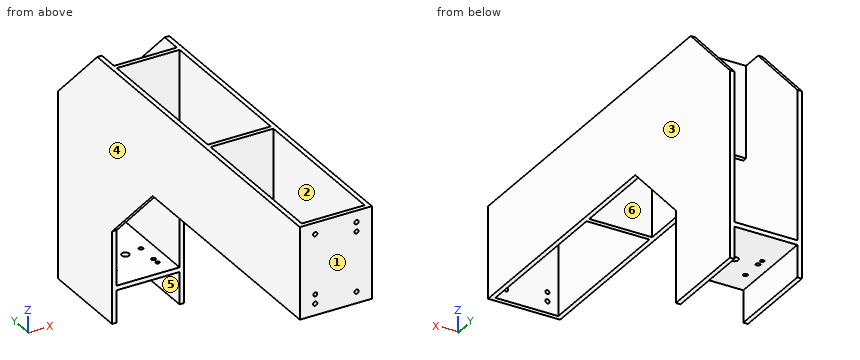
```python
from build123d import *

# Parameters (mm, degrees)
BOSS_EXTRUDE1_DEPTH      = 10
BOSS_EXTRUDE1_DEPTH_BACK = 147
SKETCH3_W                = 137
SKETCH3_H                = 550
CUT_EXTRUDE1_DEPTH       = 885
SKETCH4_W                = 137
SKETCH4_H                = 200
BOSS_EXTRUDE2_DEPTH      = 10
CUT_EXTRUDE3_REACH       = 82
SKETCH6_R                = 4.5
SKETCH6_R_2              = 8
SKETCH6_R_3              = 4.25
SKETCH8_W                = 157
SKETCH8_H                = 200
BOSS_EXTRUDE3_DEPTH      = 10
LPATTERN1_COUNT          = 3
LPATTERN1_PITCH          = 347.5
CUT_EXTRUDE4_REACH       = 12
SKETCH7_R                = 4.5
SKETCH7_R_2              = 4.25


with BuildPart() as part:
    # Sketch1 → Boss-Extrude1 (new body, two sides)
    with BuildSketch(Plane(origin=(0, 0, 0), x_dir=(0, 0, -1), z_dir=(1, 0, 0))) as boss_extrude1_sk:
        Polygon((200, 695), (200, 545), (350, 695), align=None)
        Polygon((200, 0), (200, 695), (550, 695), (550, 895), (145, 895), (0, 750), (0, 0), align=None)
    extrude(amount=BOSS_EXTRUDE1_DEPTH)
    extrude(boss_extrude1_sk.sketch, amount=-BOSS_EXTRUDE1_DEPTH_BACK)

    # Sketch3 → Cut-Extrude1 (cut)
    with BuildSketch(Plane(origin=(0, 895, 0), x_dir=(1, 0, 0), z_dir=(0, 1, 0))):
        with Locations((-68.5, 275)):
            Rectangle(SKETCH3_W, SKETCH3_H)
    extrude(amount=-CUT_EXTRUDE1_DEPTH, mode=Mode.SUBTRACT)

    # Sketch4 → Boss-Extrude2 (add)
    with BuildSketch(Plane(origin=(0, 0, -480), x_dir=(-1, 0, 0), z_dir=(0, 0, -1))):
        with Locations((68.5, 795)):
            Rectangle(SKETCH4_W, SKETCH4_H)
    extrude(amount=-BOSS_EXTRUDE2_DEPTH)

    # Sketch6 → Cut-Extrude3 (cut, up to next)
    with BuildSketch(Plane.XY.offset(-470), mode=Mode.PRIVATE) as cut_extrude3_sk1:
        with Locations((-111, 747.2)):
            Circle(SKETCH6_R)
    cut_extrude3_tool1 = extrude(cut_extrude3_sk1.sketch, amount=-CUT_EXTRUDE3_REACH, mode=Mode.PRIVATE) & part.part
    add(cut_extrude3_tool1.solids().sort_by_distance((-111, 747.2, -470))[0], mode=Mode.SUBTRACT)
    # Sketch6 → Cut-Extrude3 (cut, up to next)
    with BuildSketch(Plane.XY.offset(-470), mode=Mode.PRIVATE) as cut_extrude3_sk2:
        with Locations((-26, 747.2)):
            Circle(SKETCH6_R)
    cut_extrude3_tool2 = extrude(cut_extrude3_sk2.sketch, amount=-CUT_EXTRUDE3_REACH, mode=Mode.PRIVATE) & part.part
    add(cut_extrude3_tool2.solids().sort_by_distance((-26, 747.2, -470))[0], mode=Mode.SUBTRACT)
    # Sketch6 → Cut-Extrude3 (cut, up to next)
    with BuildSketch(Plane.XY.offset(-470), mode=Mode.PRIVATE) as cut_extrude3_sk3:
        with Locations((-111, 793.7)):
            Circle(SKETCH6_R)
    cut_extrude3_tool3 = extrude(cut_extrude3_sk3.sketch, amount=-CUT_EXTRUDE3_REACH, mode=Mode.PRIVATE) & part.part
    add(cut_extrude3_tool3.solids().sort_by_distance((-111, 793.7, -470))[0], mode=Mode.SUBTRACT)
    # Sketch6 → Cut-Extrude3 (cut, up to next)
    with BuildSketch(Plane.XY.offset(-470), mode=Mode.PRIVATE) as cut_extrude3_sk4:
        with Locations((-26, 793.7)):
            Circle(SKETCH6_R)
    cut_extrude3_tool4 = extrude(cut_extrude3_sk4.sketch, amount=-CUT_EXTRUDE3_REACH, mode=Mode.PRIVATE) & part.part
    add(cut_extrude3_tool4.solids().sort_by_distance((-26, 793.7, -470))[0], mode=Mode.SUBTRACT)
    # Sketch6 → Cut-Extrude3 (cut, up to next)
    with BuildSketch(Plane.XY.offset(-470), mode=Mode.PRIVATE) as cut_extrude3_sk5:
        with Locations((-63, 788.5)):
            Circle(SKETCH6_R_2)
    cut_extrude3_tool5 = extrude(cut_extrude3_sk5.sketch, amount=-CUT_EXTRUDE3_REACH, mode=Mode.PRIVATE) & part.part
    add(cut_extrude3_tool5.solids().sort_by_distance((-63, 788.5, -470))[0], mode=Mode.SUBTRACT)
    # Sketch6 → Cut-Extrude3 (cut, up to next)
    with BuildSketch(Plane.XY.offset(-470), mode=Mode.PRIVATE) as cut_extrude3_sk6:
        with Locations((-111, 808.7)):
            Circle(SKETCH6_R_3)
    cut_extrude3_tool6 = extrude(cut_extrude3_sk6.sketch, amount=-CUT_EXTRUDE3_REACH, mode=Mode.PRIVATE) & part.part
    add(cut_extrude3_tool6.solids().sort_by_distance((-111, 808.7, -470))[0], mode=Mode.SUBTRACT)
    # Sketch6 → Cut-Extrude3 (cut, up to next)
    with BuildSketch(Plane.XY.offset(-470), mode=Mode.PRIVATE) as cut_extrude3_sk7:
        with Locations((-26, 732.2)):
            Circle(SKETCH6_R_3)
    cut_extrude3_tool7 = extrude(cut_extrude3_sk7.sketch, amount=-CUT_EXTRUDE3_REACH, mode=Mode.PRIVATE) & part.part
    add(cut_extrude3_tool7.solids().sort_by_distance((-26, 732.2, -470))[0], mode=Mode.SUBTRACT)

    # Sketch8 → Boss-Extrude3 (add)
    with BuildSketch(Plane(origin=(0, 705, 0), x_dir=(-1, 0, 0), z_dir=(0, -1, 0))):
        with Locations((68.5, 100)):
            Rectangle(SKETCH8_W, SKETCH8_H)
    boss_extrude3 = extrude(amount=BOSS_EXTRUDE3_DEPTH)

    # LPattern1: Boss-Extrude3 ×3
    with Locations(*[(0, -i * LPATTERN1_PITCH, 0) for i in range(1, LPATTERN1_COUNT)]):
        add(boss_extrude3)

    # Sketch7 → Cut-Extrude4 (cut, up to next)
    with BuildSketch(Plane(origin=(0, 10, 0), x_dir=(1, 0, 0), z_dir=(0, 1, 0)), mode=Mode.PRIVATE) as cut_extrude4_sk1:
        with Locations((-113.5, 175)):
            Circle(SKETCH7_R)
    cut_extrude4_tool1 = extrude(cut_extrude4_sk1.sketch, amount=-CUT_EXTRUDE4_REACH, mode=Mode.PRIVATE) & part.part
    add(cut_extrude4_tool1.solids().sort_by_distance((-113.5, 10, -175))[0], mode=Mode.SUBTRACT)
    # Sketch7 → Cut-Extrude4 (cut, up to next)
    with BuildSketch(Plane(origin=(0, 10, 0), x_dir=(1, 0, 0), z_dir=(0, 1, 0)), mode=Mode.PRIVATE) as cut_extrude4_sk2:
        with Locations((-23.5, 175)):
            Circle(SKETCH7_R)
    cut_extrude4_tool2 = extrude(cut_extrude4_sk2.sketch, amount=-CUT_EXTRUDE4_REACH, mode=Mode.PRIVATE) & part.part
    add(cut_extrude4_tool2.solids().sort_by_distance((-23.5, 10, -175))[0], mode=Mode.SUBTRACT)
    # Sketch7 → Cut-Extrude4 (cut, up to next)
    with BuildSketch(Plane(origin=(0, 10, 0), x_dir=(1, 0, 0), z_dir=(0, 1, 0)), mode=Mode.PRIVATE) as cut_extrude4_sk3:
        with Locations((-23.5, 25)):
            Circle(SKETCH7_R)
    cut_extrude4_tool3 = extrude(cut_extrude4_sk3.sketch, amount=-CUT_EXTRUDE4_REACH, mode=Mode.PRIVATE) & part.part
    add(cut_extrude4_tool3.solids().sort_by_distance((-23.5, 10, -25))[0], mode=Mode.SUBTRACT)
    # Sketch7 → Cut-Extrude4 (cut, up to next)
    with BuildSketch(Plane(origin=(0, 10, 0), x_dir=(1, 0, 0), z_dir=(0, 1, 0)), mode=Mode.PRIVATE) as cut_extrude4_sk4:
        with Locations((-113.5, 25)):
            Circle(SKETCH7_R)
    cut_extrude4_tool4 = extrude(cut_extrude4_sk4.sketch, amount=-CUT_EXTRUDE4_REACH, mode=Mode.PRIVATE) & part.part
    add(cut_extrude4_tool4.solids().sort_by_distance((-113.5, 10, -25))[0], mode=Mode.SUBTRACT)
    # Sketch7 → Cut-Extrude4 (cut, up to next)
    with BuildSketch(Plane(origin=(0, 10, 0), x_dir=(1, 0, 0), z_dir=(0, 1, 0)), mode=Mode.PRIVATE) as cut_extrude4_sk5:
        with Locations((-113.5, 155)):
            Circle(SKETCH7_R_2)
    cut_extrude4_tool5 = extrude(cut_extrude4_sk5.sketch, amount=-CUT_EXTRUDE4_REACH, mode=Mode.PRIVATE) & part.part
    add(cut_extrude4_tool5.solids().sort_by_distance((-113.5, 10, -155))[0], mode=Mode.SUBTRACT)
    # Sketch7 → Cut-Extrude4 (cut, up to next)
    with BuildSketch(Plane(origin=(0, 10, 0), x_dir=(1, 0, 0), z_dir=(0, 1, 0)), mode=Mode.PRIVATE) as cut_extrude4_sk6:
        with Locations((-23.5, 45)):
            Circle(SKETCH7_R_2)
    cut_extrude4_tool6 = extrude(cut_extrude4_sk6.sketch, amount=-CUT_EXTRUDE4_REACH, mode=Mode.PRIVATE) & part.part
    add(cut_extrude4_tool6.solids().sort_by_distance((-23.5, 10, -45))[0], mode=Mode.SUBTRACT)


solid = part.part
```
Here's how the part is built. I have some questions about the finished solid (model axes, mm). Face numbers are marked on the shaded views. A direction names the side the tool comes from. Round coordinates to 2 decimals unless told otherwise and drop trailing zeros. Write each loop counter-clockwise with the first axis right and the second up, starting at its lowest first coordinate (ties: lowest second). Pieces come first, ordered by that corner, then holes.
Q1. If we mould it in two halves opening along Y, with no side actions, what happens to the marked faces 1, 2 and 3? For each: +Y half, -Y half, draft (parallel to the pull), parting line (faces both ways), or undercut.
Q2. If we section it at B-B on z = -427: Write out the boundary of the cut face in (x, y).
Q3. If we section it at D-D on z = -69: Write out the boundary of the cut face in (x, y), plus the area to 3 significant figures.
Q4. Please list where these lines run through material, in increasing order: probe 1 along Z at (x, y) = (-113, 5); probe 2 along Y at (x, z) = (-94, -131.5); probe 3 along Y at (x, z) = (-111, -477.25).
Q5. If we section it at A-A on y = 286.5: Write out the boundary of the cut face in (x, z).
Q6. If we section it at C-C on x = -91: Write out the boundary of the cut face in (y, z), plus the area to 3 significant figures.
Q7. Will these pins go through, and if not, where does the flat tip stop? P1, Ø10.5, axis at x = -111, y = 747.2, coming from the -Z side; P2, Ø5, axis at x = -26, y = 732.2, coming from the +Z side (3 decimals); P3, Ø11, axis at x = -23.5, z = -45, coming from the +Y side; P4, Ø8, axis at x = -107.5, z = -82.5, coming from the -Y side.
Q8. Which directions (+Z, -Z, +X, -X, +Y, -Y) give clear straight access to the entire face, cutting with the end or side of a thin tool? Please do the marked faces 4, 5 and 6.
Answer below:
1. face 1: -Y half
1. face 2: undercut
1. face 3: draft
2. outline: (-147, 695) - (-137, 695) - (-137, 895) - (-147, 895) - close; (0, 695) - (10, 695) - (10, 895) - (0, 895) - close
3. outline: (-147, 0) - (10, 0) - (10, 819) - (0, 819) - (0, 705) - (-137, 705) - (-137, 819) - (-147, 819) - close; hole (-137, 10) - (0, 10) - (0, 347.5) - (-137, 347.5) - close; hole (-137, 357.5) - (0, 357.5) - (0, 695) - (-137, 695) - close
3. area: 20,500 mm2
4. probe 1: z = -200 to -179.47, -170.53 to -159.22, -150.78 to -29.47, -20.53 to 0
4. probe 2: y = 0 to 10, 347.5 to 357.5, 695 to 705
4. probe 3: y = 695 to 742.7, 751.7 to 789.2, 798.2 to 804.45, 812.95 to 895
5. outline: (-147, -200) - (-137, -200) - (-137, 0) - (-147, 0) - close; (0, -200) - (10, -200) - (10, 0) - (0, 0) - close
6. outline: (0, -200) - (10, -200) - (10, 0) - (0, 0) - close; (347.5, -200) - (357.5, -200) - (357.5, 0) - (347.5, 0) - close; (695, -480) - (895, -480) - (895, -470) - (695, -470) - close; (695, -200) - (705, -200) - (705, 0) - (695, 0) - close
6. area: 8,000 mm2
7. P1: stops at z = -480
7. P2: passes through
7. P3: stops at y = 705
7. P4: stops at y = 0
8. face 4: +Z, -Z, -X, +Y, -Y
8. face 5: -Z, +Y, -Y
8. face 6: +Z, -Z
